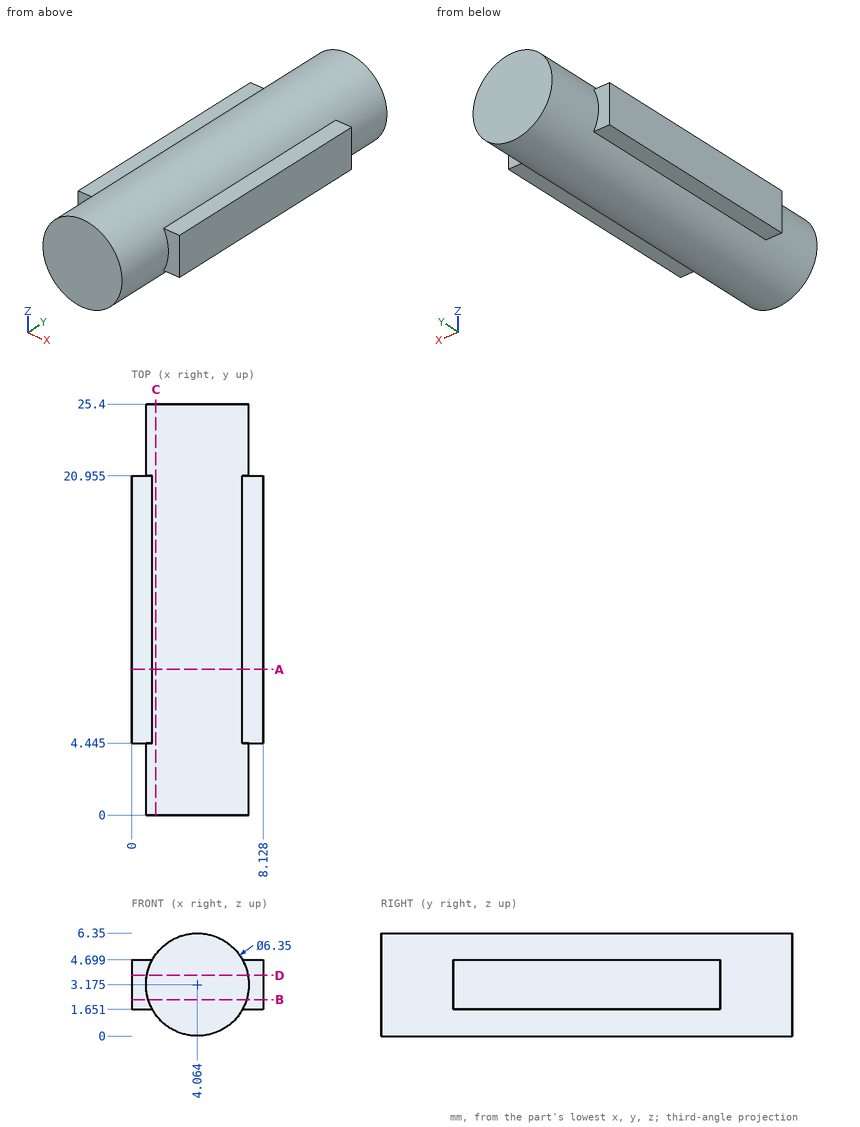
Verification items for this drawing (mm, ordinates from the low corner). Round coordinates to 2 decimals unless told otherwise and drop trailing zeros. Loops run counter-clockwise (first coordinate to the right, second up) from the corner with the lowest first, then second, coordinate; pieces in that order, holes last. Notation, with made-up numbers: (45, 69) - (102, 69) arc R17 ccw to (102, 78) - close; hole circle Ø9 at (-4, 68). An arc over 180 degrees is marked (long way). Answer as CSV lines item,"result". Start each with the question number.
Item 1: Section check B-B (z = 2.25). Record the boundary of the cut face in (x, y) (3 decimals), and give its area (3 significant figures).
Item 2: Section check A-A (y = 9). Record the boundary of the cut face in (x, z) (3 decimals).
Item 3: Section check C-C (x = 1.5). Record the boundary of the cut face in (y, z), and give its area (3 significant figures).
Item 4: Depth check by flat-ended pin: P1, Ø0.6, axis at x = 7.5, y = 13.5, coming from the +Z side; P2, Ø1, axis at x = 2.5, y = 12.5, coming from the -Z side. Enter the tip coordinate at first touch or a pass-through.
Item 5: Scan lines: line 1 (Z direction, x = 1, y = 11.5); line 2 (Y direction, x = 7.5, z = 3.75) (3 decimals); line 3 (X direction, y = 23.25, z = 6). Record each from-to range of solid material in increasing order. Write a range as [from, to].
Item 6: Section check D-D (z = 3.75). Record the boundary of the cut face in (x, y) (1 decimal), and give its area (3 significant figures).
Report:
1,outline,"(0, 4.445) - (1.027, 4.445) - (1.027, 0) - (7.101, 0) - (7.101, 4.445) - (8.128, 4.445) - (8.128, 20.955) - (7.101, 20.955) - (7.101, 25.4) - (1.027, 25.4) - (1.027, 20.955) - (0, 20.955) - close"
1,area,"188 mm2"
2,outline,"(0, 1.651) - (1.279, 1.651) arc R3.175 ccw to (6.849, 1.651) - (8.128, 1.651) - (8.128, 4.699) - (6.849, 4.699) arc R3.175 ccw to (1.279, 4.699) - (0, 4.699) - close"
3,outline,"(0, 1.3) - (25.4, 1.3) - (25.4, 5.05) - (0, 5.05) - close"
3,area,"95.1 mm2"
4,P1,"stops at z = 4.7"
4,P2,"stops at z = 0.18"
5,line 1,"z = [1.65, 4.7]"
5,line 2,"y = [4.445, 20.955]"
5,line 3,"x = [2.61, 5.51]"
6,outline,"(0, 4.4) - (0.9, 4.4) - (0.9, 0) - (7.2, 0) - (7.2, 4.4) - (8.1, 4.4) - (8.1, 21) - (7.2, 21) - (7.2, 25.4) - (0.9, 25.4) - (0.9, 21) - (0, 21) - close"
6,area,"190 mm2"
